from build123d import *

# Parameters (mm, degrees)
BOSS_EXTRU_1_DEPTH      = 70
ESQUISSE5_W             = 40
ESQUISSE5_H             = 15
ENL_V_MAT_EXTRU_2_DEPTH = 10
ESQUISSE7_W             = 15
ESQUISSE7_H             = 4
BOSS_EXTRU_4_DEPTH      = 50
ENL_V_MAT_EXTRU_6_DEPTH = 3.2
ENL_V_MAT_EXTRU_7_DEPTH = 3.2
CONG_1_R                = 6
ESQUISSE19_W            = 3
ESQUISSE19_H            = 15
BOSS_EXTRU_6_DEPTH      = 19
CONG_3_R                = 4
CONG_5_R                = 3


with BuildPart() as part:
    # Esquisse1 → Boss.-Extru.1 (new body)
    with BuildSketch(Plane.XY):
        with BuildLine():
            Line((-31.982945736, 17), (-31.982945736, 0))
            Line((-31.982945736, 0), (-16.982945736, 0))
            Line((-16.982945736, 0), (-16.982945736, 4))
            Line((-16.982945736, 4), (-24.982945736, 4))
            ThreePointArc((-24.982945736, 4), (-27.811372861, 5.171572875), (-28.982945736, 8))
            Line((-28.982945736, 8), (-28.982945736, 13))
            Line((-28.982945736, 13), (-23.982945736, 17.5))
            ThreePointArc((-23.982945736, 17.5), (-24.422285565, 18.560660172), (-25.482945736, 19))
            Line((-25.482945736, 19), (-28.982945736, 19))
            Line((-28.982945736, 19), (-29.982945736, 19))
            Line((-29.982945736, 19), (-31.982945736, 19))
            Line((-31.982945736, 19), (-31.982945736, 18))
            Line((-31.982945736, 18), (-31.982945736, 17))
        make_face()
    extrude(amount=BOSS_EXTRU_1_DEPTH)

    # Esquisse5 → Enlèv. mat.-Extru.2 (cut)
    with BuildSketch(Plane.ZY.offset(31.982945736)):
        with Locations((35, 11.5)):
            Rectangle(ESQUISSE5_W, ESQUISSE5_H)
    extrude(amount=-ENL_V_MAT_EXTRU_2_DEPTH, mode=Mode.SUBTRACT)

    # Esquisse7 → Boss.-Extru.4 (add)
    with BuildSketch(Plane(origin=(-16.982945736, 0, 0), x_dir=(0, 0, -1), z_dir=(1, 0, 0))):
        with Locations((-15.5, 2)):
            Rectangle(ESQUISSE7_W, ESQUISSE7_H)
        with Locations((-54.5, 2)):
            Rectangle(ESQUISSE7_W, ESQUISSE7_H)
    extrude(amount=BOSS_EXTRU_4_DEPTH)

    # Esquisse17 → Enlèv. mat.-Extru.6 (cut)
    with BuildSketch(Plane(origin=(0, 4, 0), x_dir=(1, 0, 0), z_dir=(0, 1, 0))):
        Polygon((5.081081476, -50.925), (0.953027051, -50.925), (-1.111000161, -54.5), (0.953027051, -58.075), (5.081081476, -58.075), (7.145108688, -54.5), align=None)
        Polygon((16.921295497, -58.056491041), (5.081081476, -58.075), (7.145108688, -54.5), (5.081081476, -50.925), (16.984922057, -50.906774147), (14.88916329, -54.463265188), align=None)
        Polygon((16.921295497, -58.056491041), (21.04918647, -58.093225853), (23.144945237, -54.536734812), (21.11281303, -50.943508959), (16.984922057, -50.906774147), (14.88916329, -54.463265188), align=None)
    extrude(amount=-ENL_V_MAT_EXTRU_6_DEPTH, mode=Mode.SUBTRACT)

    # Esquisse18 → Enlèv. mat.-Extru.7 (cut)
    with BuildSketch(Plane(origin=(0, 0.8, 0), x_dir=(1, 0, 0), z_dir=(0, 1, 0))):
        with BuildLine():
            Line((19.104945237, -52.430616368), (2.928995206, -52.406118437))
            ThreePointArc((2.928995206, -52.406118437), (0.828995206, -54.506118437), (2.928995206, -56.606118437))
            Line((2.928995206, -56.606118437), (19.104945237, -56.630616368))
            ThreePointArc((19.104945237, -56.630616368), (21.204945237, -54.530616368), (19.104945237, -52.430616368))
        make_face()
    extrude(amount=-ENL_V_MAT_EXTRU_7_DEPTH, mode=Mode.SUBTRACT)

    # Congé1
    cong_1_edges = [part.edges().sort_by_distance(p)[0] for p in [
        (-16.982945736, 2, 0),
        (-16.982945736, 2, 70),
    ]]
    fillet(cong_1_edges, radius=CONG_1_R)

    # Esquisse19 → Boss.-Extru.6 (add)
    with BuildSketch(Plane.XZ):
        with Locations((-33.482945736, 62.5)):
            Rectangle(ESQUISSE19_W, ESQUISSE19_H)
        with Locations((-33.482945736, 7.5)):
            Rectangle(ESQUISSE19_W, ESQUISSE19_H)
    extrude(amount=-BOSS_EXTRU_6_DEPTH)

    # Congé3
    cong_3_edges = [part.edges().sort_by_distance(p)[0] for p in [
        (-34.982945736, 9.5, 70),
        (-34.982945736, 9.5, 0),
    ]]
    fillet(cong_3_edges, radius=CONG_3_R)

    # Congé5
    cong_5_edges = [part.edges().sort_by_distance(p)[0] for p in [
        (-34.982945736, 9.5, 55),
        (-34.982945736, 9.5, 15),
    ]]
    fillet(cong_5_edges, radius=CONG_5_R - 0.0001)  # a hair under: the kernel refuses the full size


solid = part.part
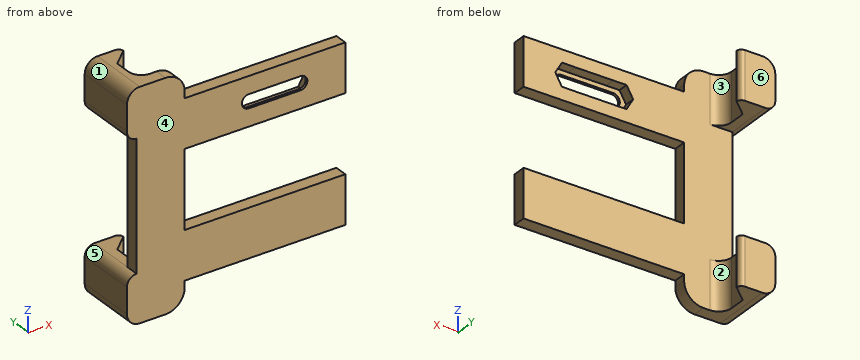
Design review of the part built by this model. Coordinates are the model's own, in mm. Face numbers are marked on the shaded views. A direction names the side the tool comes from. Give positions to 0.01 mm unless a question says otherwise; leave off trailing zeros. Loops run counter-clockwise (first coordinate to the right, second up) from the corner with the lowest first, then second, coordinate; pieces in that order, holes last. Notation, with made-up numbers: (15, 83.5) - (40, 83.5) arc R35 ccw to (40, 119.5) - close; hole circle Ø9 at (16.25, 49.5). An arc over 180 degrees is marked (long way). Use CSV: the item, a comma, the result in double quotes. Start each with the question number.
1. Insertion check: P1, Ø5.5, axis at x = 12.5, z = 55, coming from the +Y side; P2, Ø4, axis at x = -28.5, y = 8, coming from the +Z side; P3, Ø1.2, axis at x = 4.5, y = 1, coming from the +Z side; P4, Ø6, axis at y = 11.5, z = 59, coming from the +X side. Each pin has a flat end and moves straight along its axis. Give the tip position at first contact, or say it passes through.
2. Add section A-A (y = 11.25). State the section outline as (x, z) points, plus the area to 3 significant figures.
3. Wall thickness on L1, parallel to Z at x = 20, y = 1.25; L2, parallel to Z at x = -12, y = 3.25; L3, parallel to Z at x = 22.5, y = 2.25: over which ranges is each line inside the solid? List them lowest first.
4. Add section D-D (x = 14). State the section outline as (y, z) points, plus the area to 3 significant figures.
5. Machinability: for the marked faces 1 and 2, which of the approach directions +Z, -Z, +X, -X, +Y, -Y give a long, thin tool a straight path to every point of the face, cutting with its end or side? Answer none if there is none.
6. Draft analysis for pull direction Y (two halves, no side actions). For the marked faces 3, 4, 5 and 6, state which applies: released by +Y, released by -Y, zero draft, split by the parting line, or undercut.
7. Add section C-C (x = -30). State the section outline as (y, z) points.
8. Add section B-B (x = 26). State the section outline as (y, z) points.
Results found:
1,P1,"stops at y = 0.8"
1,P2,"stops at z = 70"
1,P3,"stops at z = 62"
1,P4,"stops at x = -27.32"
2,outline,"(-34.98, 4) arc R4 ccw to (-30.98, 0) - (-28.98, 0) - (-28.98, 15) - (-31.98, 15) arc R3 ccw to (-34.98, 12) - close; (-34.98, 58) arc R3 ccw to (-31.98, 55) - (-28.98, 55) - (-28.98, 70) - (-30.98, 70) arc R4 ccw to (-34.98, 66) - close"
2,area,"169 mm²"
3,L1,"z = 8 to 23, 47 to 50.93, 58.08 to 62"
3,L2,"z = 8 to 23, 47 to 62"
3,L3,"z = 8 to 23, 47 to 53.4, 55.63 to 62"
4,outline,"(0, 8) - (4, 8) - (4, 23) - (0, 23) - close; (0, 47) - (4, 47) - (4, 50.91) - (0.8, 50.91) - (0.8, 52.42) - (0, 52.42) - close; (0, 56.62) - (0.8, 56.62) - (0.8, 58.06) - (4, 58.06) - (4, 62) - (0, 62) - close"
4,area,"93.8 mm²"
5,face 1,"+Z, -X, +Y, -Y"
5,face 2,"+Z, -Z, +X"
6,face 3,"undercut"
6,face 4,"released by -Y"
6,face 5,"zero draft"
6,face 6,"released by +Y"
7,outline,"(0, 0) - (19, 0) - (19, 15) - (4, 15) - (4, 55) - (19, 55) - (19, 70) - (0, 70) - close"
8,outline,"(0, 8) - (4, 8) - (4, 23) - (0, 23) - close; (0, 47) - (4, 47) - (4, 62) - (0, 62) - close"
